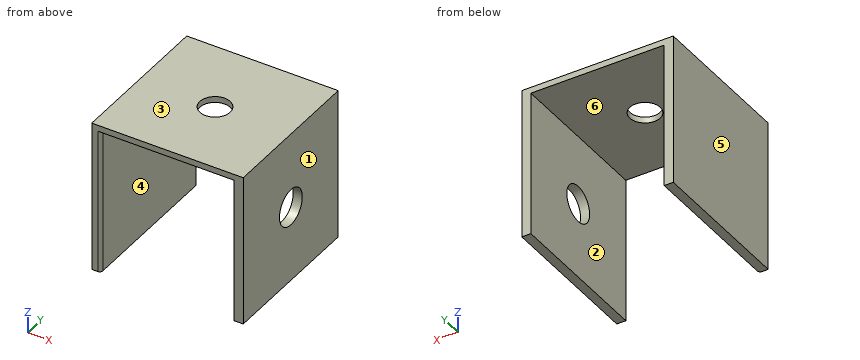
```python
from build123d import *

# Parameters (mm, degrees)
BOX003_W        = 44
BOX003_H        = 60
BOX003_DEPTH    = 50
BOX002_W        = 50
BOX002_H        = 50
BOX002_DEPTH    = 50
SKETCH002_R     = 5.003926
POCKET001_DEPTH = 58
SKETCH003_R     = 6
POCKET002_DEPTH = 5
FILLET_R        = 1


with BuildPart() as cubo003:
    # Box003 → Box003 (new body)
    with BuildSketch(Plane(origin=(117, -42, -2), x_dir=(1, 0, 0), z_dir=(0, 0, 1))):
        with Locations((22, 30)):
            Rectangle(BOX003_W, BOX003_H)
    extrude(amount=BOX003_DEPTH)


with BuildPart() as fillet_body:
    # Box002 → Box002 (new body)
    with BuildSketch(Plane(origin=(114, -39, 0), x_dir=(1, 0, 0), z_dir=(0, 0, 1))):
        with Locations((25, 25)):
            Rectangle(BOX002_W, BOX002_H)
    extrude(amount=BOX002_DEPTH)

    # Sketch002 → Pocket001 (cut)
    with BuildSketch(Plane(origin=(114, -39, 50), x_dir=(1, 0, 0), z_dir=(0, 0, 1))):
        with Locations((25, 25)):
            Circle(SKETCH002_R)
    extrude(amount=-POCKET001_DEPTH, mode=Mode.SUBTRACT)

    # Cut003: cut Cubo003
    add(cubo003.part, mode=Mode.SUBTRACT)

    # Sketch003 → Pocket002 (cut)
    with BuildSketch(Plane.YZ.offset(164)):
        with Locations((-13.931141, 25)):
            Circle(SKETCH003_R)
    extrude(amount=-POCKET002_DEPTH, mode=Mode.SUBTRACT)

    # Fillet
    fillet_edges = [fillet_body.edges().sort_by_distance(p)[0] for p in [
        (117, -39, 24),
    ]]
    fillet(fillet_edges, radius=FILLET_R)


solid = fillet_body.part
```
Could you check a few things on this model? Use its own coordinates, in mm. Face numbers are marked on the shaded views. A direction names the side the tool comes from. Give positions to 0.01 mm unless a question says otherwise; leave off trailing zeros. Order: outer loops, then holes, each group sorted by start corner. A loop starts at its lowest first (then second) coordinate and runs counter-clockwise, first axis right, second up.
Q1. Suppose I cut it at D-D, the plane y = -14. Write out the boundary of the cut face in (x, z).
Q2. Suppose I cut it at C-C, the plane z = 44. Write out the boundary of the cut face in (x, y), and give its area (3 significant figures).
Q3. Suppose I cut it at B-B, the plane z = 25. Write out the boundary of the cut face in (x, y), and give its area (3 significant figures).
Q4. I'm going to push flat-ended pins straight in: P1, Ø16, axis at x = 139, y = -14, coming from the -Z side; P2, Ø10, axis at x = 119.5, z = 30, coming from the +Y side. Where does each tip first touch, or does it pass through?
Q5. If I drill on line 1 along X through (y, z) = (9.5, 29.5); line 2 along Y through (x, z) = (139, 49.65); line 3 along Z through (x, y) = (132, -31), over which ranges is the centre line in solid material (lowest first)?
Q6. Suppose I cut it at A-A, the plane x = 139. Write out the boundary of the cut face in (y, z), and give its area (3 significant figures).
Q7. For the marked faces 1 and 2, which set-ups out of +Z, -Z, +X, -X, +Y, -Y let a thin tool reach every point of the face, with its end or its side?
Q8. We'd pull the mould along X, two halves only. Please class the marked faces 3, 4, 5 and 6: +X half, -X half, draft (parallel to the pull), parting line (faces both ways), or undercut.
Solution:
1. outline: (114, 0) - (117, 0) - (117, 48) - (134, 48) - (134, 50) - (114, 50) - close; (144, 48) - (161, 48) - (161, 31) - (164, 31) - (164, 50) - (144, 50) - close; (161, 0) - (164, 0) - (164, 19) - (161, 19) - close
2. outline: (114, -39) - (116, -39) arc R1 ccw to (117, -38) - (117, 11) - (114, 11) - close; (161, -39) - (164, -39) - (164, 11) - (161, 11) - close
2. area: 300 mm2
3. outline: (114, -39) - (116, -39) arc R1 ccw to (117, -38) - (117, 11) - (114, 11) - close; (161, -39) - (164, -39) - (164, -19.93) - (161, -19.93) - close; (161, -7.93) - (164, -7.93) - (164, 11) - (161, 11) - close
3. area: 264 mm2
4. P1: stops at z = 48
4. P2: stops at y = 11
5. line 1: x = 114 to 117, 161 to 164
5. line 2: y = -39 to -19, -9 to 11
5. line 3: z = 48 to 50
6. outline: (-39, 48) - (-19, 48) - (-19, 50) - (-39, 50) - close; (-9, 48) - (11, 48) - (11, 50) - (-9, 50) - close
6. area: 80.0 mm2
7. face 1: +Z, -Z, +X, +Y, -Y
7. face 2: -Z, +Y, -Y
8. face 3: draft
8. face 4: undercut
8. face 5: -X half
8. face 6: undercut
